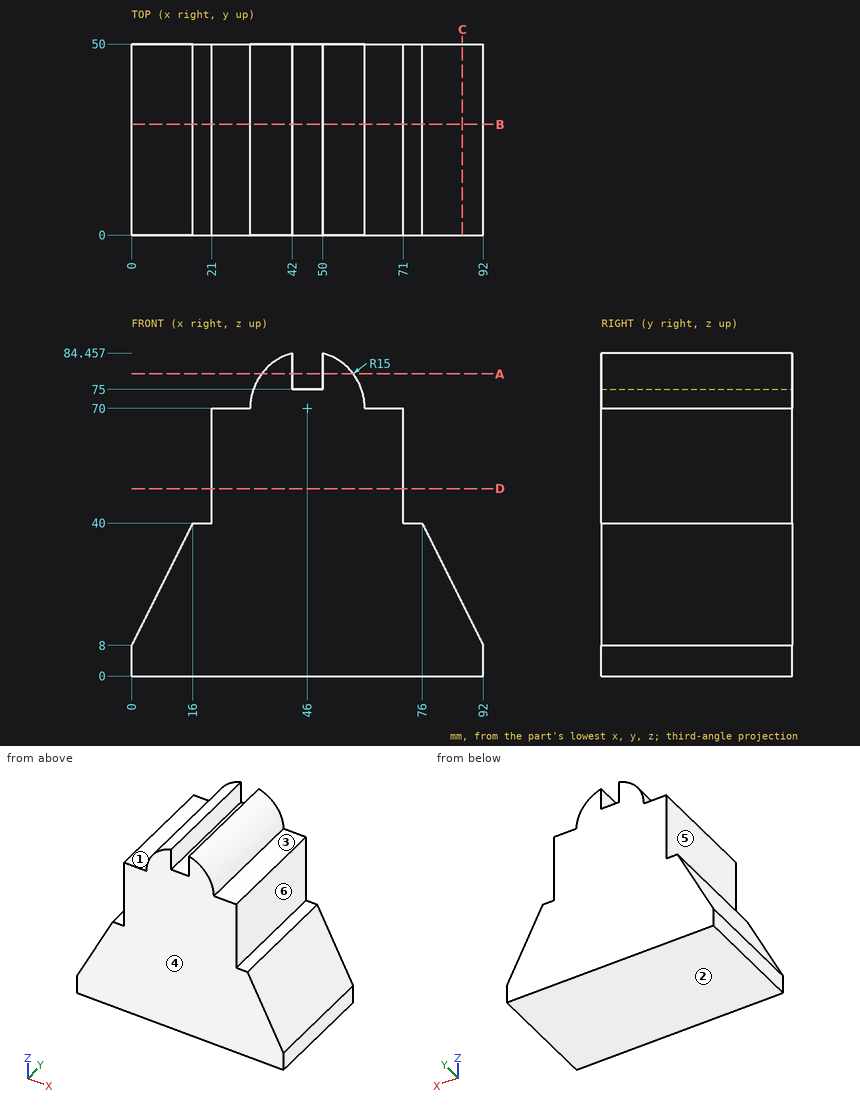
Job drawing, mm, ordinate dimensions from the low corner. One solid piece. A direction names the side the tool comes from. Coordinates: 2 decimals unless noted, no trailing zeros. Order: outer loops, then holes, each group sorted by start corner. A loop starts at its lowest first (then second) coordinate and runs counter-clockwise, first axis right, second up. Notation, with made-up numbers: (45.5, 65) - (52.5, 65) arc R17 cw to (52.5, 82) - close; hole circle Ø8 at (89, -27.75). An arc over 180 degrees is marked (long way). Return JSON: item names as keys, results as strings. Group by question number.
1) Tool access for the marked faces 1, 2 and 3: list every direction of +Z, -Z, +X, -X, +Y, -Y with a clear straight run to the whole face (end or side of a thin tool).
2) Saw through at C-C, the plane x = 86.5. Write the cut outline in (y, z), plus the area to 3 significant figures.
3) Mould opens along X. For the marked faces 4, 5 and 6 say: released by +X, released by -X, zero draft, split by the parting line, or undercut.
4) Saw through at D-D, the plane z = 49. Write the cut outline in (x, y), plus the area to 3 significant figures.
5) Saw through at B-B, the plane y = 29. Write the cut outline in (x, z), plus the area to 3 significant figures.
6) Saw through at A-A, the plane z = 79. Write the cut outline in (x, y).
7) Probe line 1 (X direction, y = 44.5, z = 56); line 2 (Z direction, x = 18, y = 15.5); line 3 (X direction, y = 19, z = 79.5). List the from-to ranges inside material, lowest first. Write a range as from..to.
8) Flat gauge pins, fed straight in: P1, Ø5, axis at x = 66, y = 29.5, coming from the +Z side; P2, Ø4.5, axis at y = 13.5, z = 81, coming from the +X side; P3, Ø8, axis at y = 32.5, z = 58.5, coming from the +X side. Where does each tip first touch, or does it go through?
Values found:
{
 "1": {"face 1": "+Z, -X, +Y, -Y", "face 2": "-Z, +X, -X, +Y, -Y", "face 3": "+Z, +X, +Y, -Y"},
 "2": {"outline": "(0, 0) - (50, 0) - (50, 19) - (0, 19) - close", "area": "950 mm²"},
 "3": {"face 4": "zero draft", "face 5": "released by -X", "face 6": "released by +X"},
 "4": {"outline": "(21, 0) - (71, 0) - (71, 50) - (21, 50) - close", "area": "2,500 mm²"},
 "5": {"outline": "(0, 0) - (92, 0) - (92, 8) - (76, 40) - (71, 40) - (71, 70) - (61, 70) arc R15 ccw to (50, 84.46) - (50, 75) - (42, 75) - (42, 84.46) arc R15 ccw to (31, 70) - (21, 70) - (21, 40) - (16, 40) - (0, 8) - close", "area": "4,940 mm²"},
 "6": {"outline": "(34, 0) - (42, 0) - (42, 50) - (34, 50) - close; (50, 0) - (58, 0) - (58, 50) - (50, 50) - close"},
 "7": {"line 1": "x = 21..71", "line 2": "z = 0..40", "line 3": "x = 34.39..42, 50..57.61"},
 "8": {"P1": "stops at z = 70", "P2": "stops at x = 58.18", "P3": "stops at x = 71"}
}
